Check sheet for the modelled part. Datum: model origin and axes. Units: mm. Round coordinates to 2 decimals unless told otherwise and drop trailing zeros. Order: outer loops, then holes, each group sorted by start corner. A loop starts at its lowest first (then second) coordinate and runs counter-clockwise, first axis right, second up.
Q1. Scan lines: probe 1 along X at (y, z) = (1.25, -10.16); probe 2 along X at (y, z) = (0.1, -121) (3 decimals); probe 3 along Z at (x, y) = (466.5, 2.2). Record each from-to range of solid material in increasing order.
Q2. Cross-section at A-A on y = 2.2. Record the cut outline in (x, z) (3 decimals), then the cut area to 3 significant figures.
Q3. Depth check by flat-ended pin: P1, Ø1, axis at y = 2, z = -128, coming from the +X side; P2, Ø10, axis at x = 521.5, z = -42.5, coming from the -Y side; P3, Ø1.6, axis at y = 1.5, z = -175, coming from the +X side; P4, Ø1.6, axis at x = 634, y = 1.5, coming from the -Z side. Enter the tip coordinate at first touch or a pass-through.
from build123d import *

# Parameters (mm, degrees)
SKETCH1_W           = 636.25984
SKETCH1_H           = 172.09262
BOSS_EXTRUDE1_DEPTH = 3.175
SKETCH2_W           = 3.175
SKETCH2_H           = 3.175
CUT_EXTRUDE1_DEPTH  = 94.36608
SKETCH3_W           = 3.175
SKETCH3_H           = 3.175
CUT_EXTRUDE5_DEPTH  = 70.49262
SKETCH4_W           = 636.25984
SKETCH4_H           = 24.39416
CUT_EXTRUDE6_DEPTH  = 660.130134708
SKETCH6_W           = 636.25984
SKETCH6_H           = 24.39416
BOSS_EXTRUDE2_DEPTH = 3.175
SKETCH7_W           = 254
SKETCH7_H           = 3.175
BOSS_EXTRUDE3_DEPTH = 6.35
SKETCH8_R           = 4.064
CUT_EXTRUDE7_DEPTH  = 661.816489847


with BuildPart() as part:
    # Sketch1 → Boss-Extrude1 (new body)
    with BuildSketch(Plane(origin=(0, 0, 0), x_dir=(1, 0, 0), z_dir=(0, 1, 0))):
        with Locations((318.12992, 86.04631)):
            Rectangle(SKETCH1_W, SKETCH1_H)
    extrude(amount=BOSS_EXTRUDE1_DEPTH)

    # Sketch2 → Cut-Extrude1 (cut)
    with BuildSketch(Plane(origin=(0, 0, -172.09262), x_dir=(-1, 0, 0), z_dir=(0, 0, -1))):
        with Locations((-318.12992, 1.5875)):
            Rectangle(SKETCH2_W, SKETCH2_H)
    extrude(amount=-CUT_EXTRUDE1_DEPTH, mode=Mode.SUBTRACT)

    # Sketch3 → Cut-Extrude5 (cut)
    with BuildSketch(Plane.XY.offset(-172.09262)):
        with Locations((1.5875, 1.5875)):
            Rectangle(SKETCH3_W, SKETCH3_H)
        with Locations((634.67234, 1.5875)):
            Rectangle(SKETCH3_W, SKETCH3_H)
    extrude(amount=CUT_EXTRUDE5_DEPTH, mode=Mode.SUBTRACT)

    # Sketch4 → Cut-Extrude6 (cut, through all)
    with BuildSketch(Plane(origin=(0, 3.175, 0), x_dir=(1, 0, 0), z_dir=(0, 1, 0))):
        with Locations((318.12992, 12.19708)):
            Rectangle(SKETCH4_W, SKETCH4_H)
    extrude(amount=-CUT_EXTRUDE6_DEPTH, mode=Mode.SUBTRACT)

    # Sketch6 → Boss-Extrude2 (add, through all)
    with BuildSketch(Plane(origin=(0, 3.175, 0), x_dir=(1, 0, 0), z_dir=(0, 1, 0))):
        with Locations((318.12992, 12.19708)):
            Rectangle(SKETCH6_W, SKETCH6_H)
    extrude(amount=-BOSS_EXTRUDE2_DEPTH)

    # Sketch7 → Boss-Extrude3 (add)
    with BuildSketch(Plane(origin=(0, 0, -172.09262), x_dir=(-1, 0, 0), z_dir=(0, 0, -1))):
        with Locations((-476.40113, 1.5875)):
            Rectangle(SKETCH7_W, SKETCH7_H)
        with Locations((-159.85871, 1.5875)):
            Rectangle(SKETCH7_W, SKETCH7_H)
    extrude(amount=BOSS_EXTRUDE3_DEPTH)

    # Sketch8 → Cut-Extrude7 (cut, through all)
    with BuildSketch(Plane(origin=(0, 3.175, 0), x_dir=(1, 0, 0), z_dir=(0, 1, 0))):
        with Locations(Location((26.107106781, 10.16, 0), (0, 0, 270))):
            Circle(SKETCH8_R)
        with Locations(Location((172.118513391, 10.16, 0), (0, 0, 270))):
            Circle(SKETCH8_R)
        with Locations(Location((318.12992, 10.16, 0), (0, 0, 270))):
            Circle(SKETCH8_R)
        with Locations(Location((464.141326609, 10.16, 0), (0, 0, 270))):
            Circle(SKETCH8_R)
        with Locations(Location((610.152733219, 10.16, 0), (0, 0, 270))):
            Circle(SKETCH8_R)
    extrude(amount=-CUT_EXTRUDE7_DEPTH, mode=Mode.SUBTRACT)


solid = part.part
Results found:
1. probe 1: x = 0 to 22.04, 30.17 to 168.05, 176.18 to 314.07, 322.19 to 460.08, 468.21 to 606.09, 614.22 to 636.26
1. probe 2: x = 3.175 to 316.542, 319.717 to 633.085
1. probe 3: z = -178.44 to -13.47, -6.85 to 0
2. outline: (0, -101.6) - (3.175, -101.6) - (3.175, -172.093) - (32.859, -172.093) - (32.859, -178.443) - (286.859, -178.443) - (286.859, -172.093) - (316.542, -172.093) - (316.542, -77.727) - (319.717, -77.727) - (319.717, -172.093) - (349.401, -172.093) - (349.401, -178.443) - (603.401, -178.443) - (603.401, -172.093) - (633.085, -172.093) - (633.085, -101.6) - (636.26, -101.6) - (636.26, 0) - (0, 0) - close; hole circle Ø8.128 at (26.107, -10.16); hole circle Ø8.128 at (172.119, -10.16); hole circle Ø8.128 at (318.13, -10.16); hole circle Ø8.128 at (464.141, -10.16); hole circle Ø8.128 at (610.153, -10.16)
2. area: 112,000 mm2
3. P1: stops at x = 633.08
3. P2: stops at y = 0
3. P3: stops at x = 603.4
3. P4: stops at z = -101.6
